The listing builds one solid part. Answer for the finished solid, in the listing's coordinates (mm). Round coordinates to 2 decimals unless told otherwise and drop trailing zeros. Loops run counter-clockwise (first coordinate to the right, second up) from the corner with the lowest first, then second, coordinate; pieces in that order, holes last. Notation, with made-up numbers: (48, 61.25) - (105, 61.25) arc R16 ccw to (105, 90.25) - close; hole circle Ø5 at (79.25, 81.5). An arc over 180 degrees is marked (long way). Write item = value, one per line. Start each with the question number.
1) For a pull along Y with two mould halves and no side action, classify faces 1 (the flat face through (13, 9, 0)), 2 (the flat face through (-110.264, 9.017, 1.972)), 3 (the cylindrical face through (88.77, 3.52, 1.97)) as released by +Y, released by -Y, zero draft, split by the parting line, or undercut.
2) Straight lines are drawn through the part: line 1 along X through (y, z) = (11, 1.35); line 2 along Y through (x, z) = (-13.5, 3.3); line 3 along X through (y, z) = (-22.5, 2.8). For each, find the intervals that lie inside material, in ascending order.
3) Section A-A, the plane y = 1.72 is taken. Determine the outline of the cut face in (x, z).
4) Section B-B, the plane z = 1.1 is taken. Give the number of separate pieces and of enclosed holes in the cut face, and give its area (3 significant figures).
5) Given pin 1 Ø2 at (x, z) = (153.5, 1.5) entering from +Y; pin 2 Ø2 at (y, z) = (42.5, 3) entering from -X; pin 3 Ø2.5 at (x, y) = (-47.17, -13.85) entering from -Z; pin 4 Ø1.5 at (x, z) = (115, 0.5) entering from +Y, each flat-ended and moving along its own axis, determine where each tip first touches the part or whether it passes through.
from build123d import *

# Parameters (mm, degrees)
SKETCH1_R           = 6
SKETCH1_R_2         = 1.15
SKETCH1_R_3         = 1.5
SKETCH1_R_4         = 2.15
SKETCH1_W           = 41.3
SKETCH1_H           = 4.35
BOSS_EXTRUDE1_DEPTH = 4
FILLET1_R           = 3


with BuildPart() as part:
    # Sketch1 → Boss-Extrude1 (new body)
    with BuildSketch(Plane.XY):
        Polygon((-128.17175976, -30), (151.82824024, -30), (151.82824024, -10), (158.82824024, -10), (158.82824024, 5), (158.82824024, 20), (151.82824024, 20), (151.82824024, 40), (67.43395693, 40), (67.43395693, 47), (37.43395693, 47), (37.43395693, 40), (-7.56604307, 40), (-7.56604307, 47), (-37.56604307, 47), (-37.56604307, 40), (-92.37604307, 40), (-128.17175976, -22), align=None)
        with Locations((-71.175741186, 1.72)):
            Circle(SKETCH1_R, mode=Mode.SUBTRACT)
        with Locations((-71.175741186, 10.22)):
            Circle(SKETCH1_R_2, mode=Mode.SUBTRACT)
        with Locations((-63.814525254, -2.53)):
            Circle(SKETCH1_R_2, mode=Mode.SUBTRACT)
        with Locations((-78.536957118, -2.53)):
            Circle(SKETCH1_R_2, mode=Mode.SUBTRACT)
        with Locations((83.04824024, 1.72)):
            Circle(SKETCH1_R, mode=Mode.SUBTRACT)
        with Locations((83.04824024, 10.22)):
            Circle(SKETCH1_R_2, mode=Mode.SUBTRACT)
        with Locations((90.409456172, -2.53)):
            Circle(SKETCH1_R_2, mode=Mode.SUBTRACT)
        with Locations((75.687024308, -2.53)):
            Circle(SKETCH1_R_2, mode=Mode.SUBTRACT)
        with Locations((92.86036, 29.5)):
            Circle(SKETCH1_R_3, mode=Mode.SUBTRACT)
        with Locations((-50.17175976, 35.5)):
            Circle(SKETCH1_R_4, mode=Mode.SUBTRACT)
        with Locations((21.82824024, 35.5)):
            Circle(SKETCH1_R_4, mode=Mode.SUBTRACT)
        with Locations((101.32824024, 35.5)):
            Circle(SKETCH1_R_4, mode=Mode.SUBTRACT)
        with Locations((-47.17175976, -13.85)):
            Circle(SKETCH1_R_3, mode=Mode.SUBTRACT)
        with Locations((2.77824024, -24.025)):
            Rectangle(SKETCH1_W, SKETCH1_H, mode=Mode.SUBTRACT)
    extrude(amount=BOSS_EXTRUDE1_DEPTH)

    # Fillet1
    fillet1_edges = [part.edges().sort_by_distance(p)[0] for p in [
        (-128.17175976, -22, 2),
        (-92.37604307, 40, 2),
        (-37.56604307, 47, 2),
        (-7.56604307, 47, 2),
        (37.43395693, 47, 2),
        (67.43395693, 47, 2),
        (151.82824024, 40, 2),
        (158.82824024, 20, 2),
        (158.82824024, -10, 2),
        (151.82824024, -30, 2),
        (-128.17175976, -30, 2),
    ]]
    fillet(fillet1_edges, radius=FILLET1_R)


solid = part.part
Geometry check:
q1.face_1 = zero draft
q1.face_2 = released by +Y
q1.face_3 = undercut
q2.line_1 = -109.12 to -72.02, -70.33 to 82.2, 83.89 to 158.83
q2.line_2 = -30 to -26.2, -21.85 to 47
q2.line_3 = -128.16 to -17.87, 23.43 to 151.83
q3.outline = (-114.48, 0) - (-77.18, 0) - (-77.18, 4) - (-114.48, 4) - close; (-65.18, 0) - (77.05, 0) - (77.05, 4) - (-65.18, 4) - close; (89.05, 0) - (158.83, 0) - (158.83, 4) - (89.05, 4) - close
q4.separate_pieces = 1
q4.enclosed_holes = 14
q4.area = 18,600 mm2
q5.pin_1 = 20
q5.pin_2 = -37.57
q5.pin_3 = through
q5.pin_4 = 40
